from build123d import *

# Parameters (mm, degrees)
SALIENTE_EXTRUIR2_DEPTH          = 160
TALADRO_DE_MARGEN_PARA_M61_D     = 6.6
TALADRO_DE_MARGEN_PARA_M61_DEPTH = 22
TALADRO_DE_MARGEN_PARA_M61_TIP   = 1.982840043


with BuildPart() as part:
    # Croquis3 → Saliente-Extruir2 (new, symmetric)
    with BuildSketch(Plane.XY):
        Polygon((-344.53, -161.11), (344.53, -161.11), (344.53, 0), (171.324919243, 100), (-405.64, 100), (-505.64, 0), align=None)
    extrude(amount=SALIENTE_EXTRUIR2_DEPTH, both=True)

    # Taladro de margen para M61
    with Locations(Plane(origin=(0, 100, 0), x_dir=(1, 0, 0), z_dir=(0, 1, 0))):
        with Locations((-67.795, 137.645), (67.795, 137.645), (-67.795, -137.645), (67.795, -137.645)):
            Hole(TALADRO_DE_MARGEN_PARA_M61_D / 2, depth=TALADRO_DE_MARGEN_PARA_M61_DEPTH)
            with Locations((0, 0, -(TALADRO_DE_MARGEN_PARA_M61_DEPTH + TALADRO_DE_MARGEN_PARA_M61_TIP / 2))):  # 118° drill point
                Cone(0, TALADRO_DE_MARGEN_PARA_M61_D / 2, TALADRO_DE_MARGEN_PARA_M61_TIP, mode=Mode.SUBTRACT)


solid = part.part
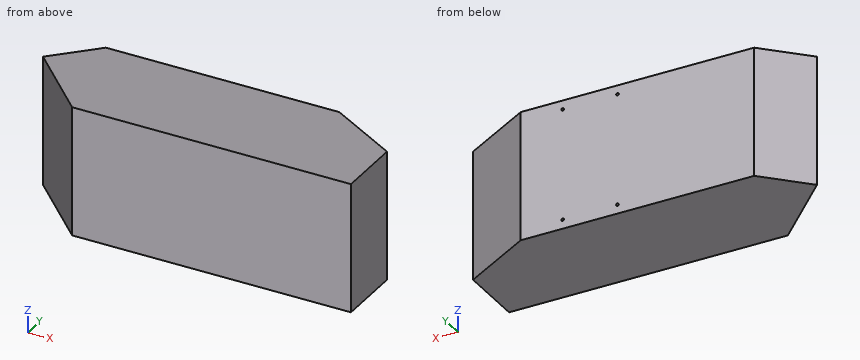
Can you work these out from the model? Positions are in its coordinate system, mm. Coordinates: 2 decimals unless noted, no trailing zeros. Write each loop counter-clockwise with the first axis right and the second up, starting at its lowest first coordinate (ties: lowest second). Pieces come first, ordered by that corner, then holes. Notation, with made-up numbers: (-4.5, -16) -> (45.5, -16) arc R20 ccw to (45.5, -2) -> close; hole circle Ø9 at (2.25, 16). An arc over 180 degrees is marked (long way). Write each question's results on one line, items separated by ' | '. Start each with the question number.
Q1. If I drill on probe 1 along X at (y, z) = (-100, -19.5); probe 2 along X at (y, z) = (-131.5, 109); probe 3 along Y at (x, z) = (295, -58), over which ranges is the centre line in solid material (lowest first)?
Q2. Imagine slicing it at A-A (z = 99). Write out the boundary of the cut face in (x, y).
Q3. Imagine slicing it at B-B (x = -431). Write out the boundary of the cut face in (y, z).
Q4. I'm going to push flat-ended pins straight in: pin 1 (1.5 mm diameter, centred on y = -58.5, z = -55.5, fed in from -X); pin 2 (1.5 mm diameter, centred on y = 70, z = -27, fed in from -X); pin 3 (12 mm diameter, centred on y = 37, z = -88, fed in from +X). Where does each tip first touch, or does it pass through?
Q5. Imagine slicing it at C-C (y = -136). Write out the boundary of the cut face in (x, z).
Taken from the geometry:
1) probe 1: x = -405.64 to 344.53 | probe 2: x = -374.14 to 344.53 | probe 3: y = -161.11 to 28.6
2) outline: (-505.64, 0) -> (-344.53, -161.11) -> (344.53, -161.11) -> (344.53, 0) -> (171.32, 100) -> (-405.64, 100) -> close
3) outline: (-74.64, -160) -> (74.64, -160) -> (74.64, 160) -> (-74.64, 160) -> close
4) pin 1: stops at x = -447.89 | pin 2: stops at x = -436.39 | pin 3: stops at x = 290.84
5) outline: (-369.64, -160) -> (344.53, -160) -> (344.53, 160) -> (-369.64, 160) -> close
